Check sheet for the modelled part. Datum: model origin and axes. Units: mm. A direction names the side the tool comes from. Round coordinates to 2 decimals unless told otherwise and drop trailing zeros. Write each loop counter-clockwise with the first axis right and the second up, starting at its lowest first coordinate (ties: lowest second). Pieces come first, ordered by that corner, then holes.
Item 1: Tool access check on faces 4 (the flat face through (308, 3, -38.1)), 5 (the flat face through (0, 3, -57)), 6 (the flat face through (-3, 3, -12.7)). Record the directions out of +Z, -Z, +X, -X, +Y, -Y that give a thin tool (end or side, any length) a straight path to the whole face; none if there is none.
Item 2: Cross-section at D-D on x = 117.5. Enter the section's corners in (y, z), plus the area to 3 significant figures.
Item 3: Cross-section at C-C on z = -6. Enter the section's corners in (x, y), plus the area to 3 significant figures.
Item 4: Material ranges on line 1 (Z direction, x = 134, y = 4.25) (3 decimals); line 2 (X direction, y = 1.25, z = -33.5); line 3 (Z direction, x = 156, y = 2.5) (3 decimals), recorded low to high.
Item 5: Go/stop test with flat-tipped pins: pin 1 Ø3 at (y, z) = (4.5, -34.5) entering from -X; pin 2 Ø1.9 at (x, y) = (-4, 3) entering from +Z; pin 3 Ø1.9 at (y, z) = (3, -30) entering from +X. Record where each tip stops, or that it passes through.
Item 6: Cross-section at A-A on x = 154.5. Enter the section's corners in (y, z) (3 decimals).
Item 7: Release check for a two-part mould opening along Z. For faces 1 (the flat face through (233, 3, -63.5)), 2 (the flat face through (0, 3, -32)), 3 (the flat face through (311.15, 3, -44)) record: +Z half, -Z half, draft (parallel to the pull), parting line (faces both ways), or undercut.
Item 8: Cross-section at B-B on z = -35. Enter the section's corners in (x, y).
from build123d import *

# Parameters (mm, degrees)
BOSS_EXTRUDE1_DEPTH = 6.35


with BuildPart() as part:
    # Sketch1 → Boss-Extrude1 (new body)
    with BuildSketch(Plane(origin=(0, 0, 0), x_dir=(1, 0, 0), z_dir=(0, 1, 0))):
        Polygon((0, 0), (146.05, 0), (146.05, -6.35), (158.75, -6.35), (158.75, 0), (304.8, 0), (304.8, 12.7), (311.15, 12.7), (311.15, 25.4), (304.8, 25.4), (304.8, 38.1), (311.15, 38.1), (311.15, 50.8), (304.8, 50.8), (304.8, 63.5), (158.75, 63.5), (158.75, 69.85), (146.05, 69.85), (146.05, 63.5), (0, 63.5), (0, 50.8), (-6.35, 50.8), (-6.35, 38.1), (0, 38.1), (0, 25.4), (-6.35, 25.4), (-6.35, 12.7), (0, 12.7), align=None)
        Polygon((132.55625, 22.225), (132.55625, 41.275), (172.24375, 41.275), (172.24375, 38.1), (184.94375, 38.1), (184.94375, 25.4), (172.24375, 25.4), (172.24375, 22.225), align=None, mode=Mode.SUBTRACT)
    extrude(amount=BOSS_EXTRUDE1_DEPTH)


solid = part.part
Response values:
1. face 4: +X, +Y, -Y
1. face 5: -Z, -X, +Y, -Y
1. face 6: +Z, -X, +Y, -Y
2. outline: (0, -63.5) - (6.35, -63.5) - (6.35, 0) - (0, 0) - close
2. area: 403 mm2
3. outline: (0, 0) - (304.8, 0) - (304.8, 6.35) - (0, 6.35) - close
3. area: 1,940 mm2
4. line 1: z = -63.5 to -41.275, -22.225 to 0
4. line 2: x = 0 to 132.56, 184.94 to 304.8
4. line 3: z = -69.85 to -41.275, -22.225 to 6.35
5. pin 1: stops at x = 0
5. pin 2: stops at z = -12.7
5. pin 3: stops at x = 304.8
6. outline: (0, -69.85) - (6.35, -69.85) - (6.35, -41.275) - (0, -41.275) - close; (0, -22.225) - (6.35, -22.225) - (6.35, 6.35) - (0, 6.35) - close
7. face 1: -Z half
7. face 2: undercut
7. face 3: draft
8. outline: (0, 0) - (132.56, 0) - (132.56, 6.35) - (0, 6.35) - close; (184.94, 0) - (304.8, 0) - (304.8, 6.35) - (184.94, 6.35) - close
